Design review of the part built by this model. Coordinates are the model's own, in mm. Face numbers are marked on the shaded views. Give positions to 0.01 mm unless a question says otherwise; leave off trailing zeros. Loops run counter-clockwise (first coordinate to the right, second up) from the corner with the lowest first, then second, coordinate; pieces in that order, holes last. Notation, with made-up numbers: (-9.5, -15.75) - (29.5, -15.75) arc R12 ccw to (29.5, -11.75) - close; hole circle Ø5 at (74, -2.5). An arc over 180 degrees is marked (long way). One line per item, written item: value. Start each with the question number.
```python
from build123d import *

# Parameters (mm, degrees)
F0_R     = 4
F1_DEPTH = 1.5
F2_R     = 1.5
F3_DEPTH = 1.9
F5_DEPTH = 1.9
F7_DEPTH = 0.3
F8_R     = 0.5


# Not quite as in the source:
# - a feature names something its author has since deleted; it is built from what else it names


with BuildPart() as f1:
    # F0 (on Top) → F1 (new body)
    with BuildSketch(Plane.XY):
        Circle(F0_R)
    extrude(amount=F1_DEPTH)

    # F2 (on face) → F3 (join)
    with BuildSketch(Plane.XY.offset(1.5)):
        Circle(F2_R)
    extrude(amount=F3_DEPTH)

    # F4 (on face) → F5 (cut)
    with BuildSketch(Plane.XY.offset(3.4)):
        with BuildLine():
            ThreePointArc((-0.4, -1.4456832295), (0, -1.5), (0.4, -1.4456832295))
            Line((0.4, -1.4456832295), (0.4, 1.4456832295))
            ThreePointArc((0.4, 1.4456832295), (0, 1.5), (-0.4, 1.4456832295))
            Line((-0.4, 1.4456832295), (-0.4, -1.4456832295))
        make_face()
        with BuildLine():
            ThreePointArc((-0.4, 1.4456832295), (0, 1.5), (0.4, 1.4456832295))
            Line((0.4, 1.4456832295), (0.4, 2.5026321411))
            Line((0.4, 2.5026321411), (-0.4, 2.5026321411))
            Line((-0.4, 2.5026321411), (-0.4, 1.4456832295))
        make_face()
    extrude(amount=-F5_DEPTH, mode=Mode.SUBTRACT)

    # F6 (on face) → F7 (join)
    with BuildSketch(Plane.XY.offset(1.5)):
        with BuildLine():
            ThreePointArc((0.4, 1.3937359865), (1.1581234822, 0.8724964183), (1.45, 0))
            ThreePointArc((1.45, 0), (1.1581234822, -0.8724964183), (0.4, -1.3937359865))
            Line((0.4, -1.3937359865), (0.4, -1.4456832295))
            ThreePointArc((0.4, -1.4456832295), (1.5, 0), (0.4, 1.4456832295))
            Line((0.4, 1.4456832295), (0.4, 1.3937359865))
        make_face()
        with BuildLine():
            ThreePointArc((-0.4, -1.3937359865), (-1.45, 0), (-0.4, 1.3937359865))
            Line((-0.4, 1.3937359865), (-0.4, 1.4456832295))
            ThreePointArc((-0.4, 1.4456832295), (-1.5, 0), (-0.4, -1.4456832295))
            Line((-0.4, -1.4456832295), (-0.4, -1.3937359865))
        make_face()
    extrude(amount=F7_DEPTH)

    # F8
    f8_edges = [f1.edges().sort_by_distance(p)[0] for p in [
        (-4, 0, 0),
    ]]
    fillet(f8_edges, radius=F8_R)


solid = f1.part
```
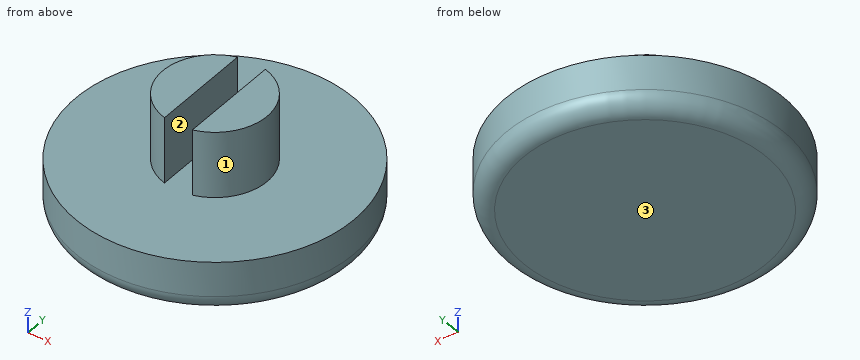
(1) Draft analysis for pull direction X (two halves, no side actions). For the marked faces 1, 2 and 3, state which applies: pulls with the +X half, pulls with the -X half, needs draft (parallel to the pull), parting line crosses it, or undercut.
(2) Take a section at B-B on x = 0. State the section outline as (y, z) points, and give its area (3 significant figures).
(3) To check wall thickness, follow L1, parallel to X at y = 1, z = 2.4; L2, parallel to X at y = 1.25, z = 3; L3, parallel to Z at x = -2, y = 0. State the ranges of each line that lie inside material, in increasing order. Write a range as from..to.
(4) Take a section at C-C on z = 0.7. State the section outline as (x, y) points.
(5) Take a section at A-A on y = 0. State the section outline as (x, z) points, and give its area (3 significant figures).
(6) For pin 1 Ø0.6 at (y, z) = (-0.5, 2.5) entering from -X; pin 2 Ø0.6 at (y, z) = (-0.5, 2.5) entering from +X; pin 3 Ø4 at (x, y) = (0.5, 2.5) entering from +Z, all flat-tipped, find the tip position at first contact; note any pin that passes through.
Here are the results:
1. face 1: pulls with the +X half
1. face 2: undercut
1. face 3: needs draft
2. outline: (-4, 0.5) arc R0.5 ccw to (-3.5, 0) - (3.5, 0) arc R0.5 ccw to (4, 0.5) - (4, 1.5) - (-4, 1.5) - close
2. area: 11.9 mm²
3. L1: -1.12..-0.4, 0.4..1.12
3. L2: -0.83..-0.4, 0.4..0.83
3. L3: 0..1.5
4. outline: circle Ø8 at (0, 0)
5. outline: (-4, 0.5) arc R0.5 ccw to (-3.5, 0) - (3.5, 0) arc R0.5 ccw to (4, 0.5) - (4, 1.5) - (1.5, 1.5) - (1.5, 3.4) - (0.4, 3.4) - (0.4, 1.5) - (-0.4, 1.5) - (-0.4, 3.4) - (-1.5, 3.4) - (-1.5, 1.5) - (-4, 1.5) - close
5. area: 16.1 mm²
6. pin 1: x = -1.49
6. pin 2: x = 1.49
6. pin 3: z = 3.4
